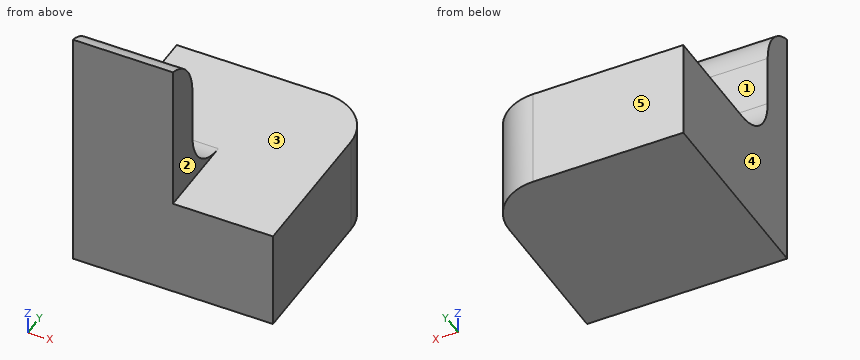
from build123d import *

# Parameters (mm, degrees)
SKETCH1_W           = 20
SKETCH1_H           = 7.5
BOSS_EXTRUDE1_DEPTH = 30
SKETCH2_W           = 40
SKETCH2_H           = 40
BOSS_EXTRUDE2_DEPTH = 20
FILLET1_R           = 10


with BuildPart() as part:
    # Sketch1 → Boss-Extrude1 (new body)
    with BuildSketch(Plane.XY):
        with Locations((-20, -3.75)):
            Rectangle(SKETCH1_W, SKETCH1_H)
    extrude(amount=BOSS_EXTRUDE1_DEPTH)

    # Sketch2 → Boss-Extrude2 (add)
    with BuildSketch(Plane.XY):
        with Locations((-10, 12.5)):
            Rectangle(SKETCH2_W, SKETCH2_H)
    extrude(amount=-BOSS_EXTRUDE2_DEPTH)

    # Fillet1
    # the kernel refuses this fillet: 10 mm, written as the material it adds along each edge
    with BuildSketch(Plane(origin=(-10, 0, 0), x_dir=(0, 1, 0), z_dir=(-1, 0, 0))) as fillet1_piece_1:
        with BuildLine():
            CenterArc((FILLET1_R, -FILLET1_R), FILLET1_R, 90, 90)
            Line((0, -FILLET1_R), (0, 0))
            Line((0, 0), (FILLET1_R, 0))
        make_face()
    extrude(amount=20)
    # the kernel refuses this fillet: 10 mm, written as the material it takes off along each edge
    with BuildSketch(Plane(origin=(10, 32.5, 25), x_dir=(-1, 0, 0), z_dir=(0, 0, -1))) as fillet1_2_piece_1:
        with BuildLine():
            CenterArc((FILLET1_R, -FILLET1_R), FILLET1_R, 90, 90)
            Line((0, -FILLET1_R), (0, 0))
            Line((0, 0), (FILLET1_R, 0))
        make_face()
    extrude(amount=70, mode=Mode.SUBTRACT)
    with BuildSketch(Plane(origin=(14.206145914, 0, 30), x_dir=(0, 0, -1), z_dir=(-1, 0, 0))) as fillet1_2_piece_2:
        with BuildLine():
            CenterArc((9.682458366, 10), FILLET1_R, 194.477512186, 75.522487814)
            Line((0, 7.5), (0, 0))
            Line((0, 0), (9.682458366, 0))
        make_face()
    extrude(amount=68.412291828, mode=Mode.SUBTRACT)


solid = part.part
For this review, take the finished solid that the model builds, in its own axes (mm). Face numbers are marked on the shaded views. A direction names the side the tool comes from. Give positions to 0.01 mm unless a question says otherwise; leave off trailing zeros. Order: outer loops, then holes, each group sorted by start corner. A loop starts at its lowest first (then second) coordinate and runs counter-clockwise, first axis right, second up. Notation, with made-up numbers: M 53.25,-37.5 L 91.25,-37.5 A19 cw 91.25,-9.5 Z; hole C 40,-30.75 d8. An arc over 180 degrees is marked long. Answer in a Markdown table with one row per item. Add a question column.
(1) For the marked faces 1, 2, 3, 4 and 5, list the 3-axis set-ups (+Z, -Z, +X, -X, +Y, -Y) from which the entire face can be reached by the end or side of a thin tool; tool diameter is ignored.
(2) Consider section D-D on y = 8. State the section outline as (x, z) points, and give its area (3 significant figures).
(3) Consider section B-B on z = 13. State the section outline as (x, y) points, and give its area (3 significant figures).
(4) For pin 1 (3 mm diameter, centred on x = -25, z = 12.5, fed in from +Y); pin 2 (20 mm diameter, centred on x = -20, y = 17, fed in from +Z); pin 3 (6 mm diameter, centred on y = 27, z = 5.5, fed in from +X); pin 4 (5 mm diameter, centred on y = -1, z = 13, fed in from +X), all flat-tipped, find the tip position at first contact; note any pin that passes through.
(5) Wall thickness on probe 1 along Z at (x, y) = (-2, -5); probe 2 along Y at (x, z) = (-27, 14); probe 3 along X at (y, z) = (-3.5, 22): over which ranges is each line inside the solid? List them lowest first. Write a range as [from, to].
(6) Consider section A-A on x = -24. State the section outline as (y, z) points.
(7) Consider section C-C on y = 17.5. State the section outline as (x, z) points.
Evaluation:
| question | item | result |
|---|---|---|
| 1 | face 1 | +Z, +X, -X, +Y |
| 1 | face 2 | +Z, +X, +Y, -Y |
| 1 | face 3 | +Z, +X, +Y |
| 1 | face 4 | +Z, -Z, -X, +Y, -Y |
| 1 | face 5 | +Z, -Z, +X, -X, +Y |
| 2 | outline | M -30,-20 L 10,-20 L 10,0 L -10,0 L -10,0.2 L -30,0.2 Z |
| 2 | area | 804 mm^2 |
| 3 | outline | M -30,-7.5 L -10,-7.5 L -10,0 L -30,0 Z |
| 3 | area | 150 mm^2 |
| 4 | pin 1 | stops at y = 0 |
| 4 | pin 2 | stops at z = 0.46 |
| 4 | pin 3 | passes through |
| 4 | pin 4 | stops at x = -10 |
| 5 | probe 1 | z = [-20, 0] |
| 5 | probe 2 | y = [-7.5, 0] |
| 5 | probe 3 | x = [-30, -10] |
| 6 | outline | M -7.5,-20 L 32.5,-20 L 32.5,0 L 10,0 A10 cw 0,10 L 0,20.32 A10 ccw -7.5,30 Z |
| 7 | outline | M -30,-20 L 10,-20 L 10,0 L -30,0 Z |
